Source: CAD feature listing. Evaluate the final solid. Frame: model axes, mm. Face numbers are marked on the shaded views. A direction names the side the tool comes from. Give positions to 0.01 mm unless a question says otherwise; leave off trailing zeros. Write each loop counter-clockwise with the first axis right and the second up, starting at its lowest first coordinate (ties: lowest second). Pieces come first, ordered by that corner, then holes. Notation, with made-up numbers: (-32, 84.25) -> (-12, 84.25) arc R26 ccw to (-12, 122.25) -> close; hole circle Ø10 at (-10, 84.5). An arc over 180 degrees is marked (long way). Use a Markdown table: item, result. Add a question column.
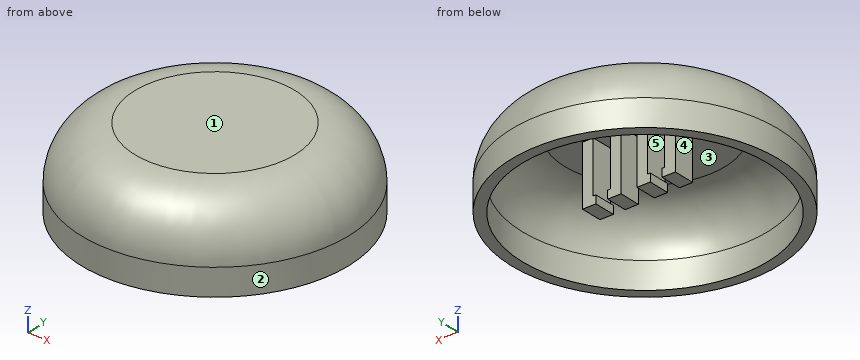
```python
from build123d import *

# Parameters (mm, degrees)
F0_R      = 31.75
F1_DEPTH  = 19.05
F2_R      = 12.7
F3_T      = -2.54
F5_W      = 2.54
F5_H      = 5.08
F6_DEPTH  = 14.224
F7_W      = 5.08
F7_H      = 1.905
F8_DEPTH  = 0.635
F9_W      = 5.08
F9_H      = 1.905
F10_DEPTH = 0.635
F11_W     = 5.08
F11_H     = 1.905
F12_DEPTH = 0.635
F13_W     = 5.08
F13_H     = 1.905
F14_DEPTH = 0.635


with BuildPart() as f1:
    # F0 (on Top) → F1 (new body)
    with BuildSketch(Plane.XY):
        Circle(F0_R)
    extrude(amount=F1_DEPTH)

    # F2
    f2_edges = [f1.edges().sort_by_distance(p)[0] for p in [
        (-31.75, 0, 19.05),
    ]]
    fillet(f2_edges, radius=F2_R)

    # F3
    f3_openings = [f1.faces().sort_by_distance(p)[0] for p in [
        (0, 0, 0),
    ]]
    offset(amount=F3_T, openings=f3_openings)

    # F5 (on face) → F6 (join)
    with BuildSketch(Plane(origin=(0, 0, 16.51), x_dir=(1, 0, 0), z_dir=(0, 0, -1))):
        with Locations((9.449818, -2.54)):
            Rectangle(F5_W, F5_H)
        with Locations((2.845818, -2.54)):
            Rectangle(F5_W, F5_H)
        with Locations((-3.48516, -2.54)):
            Rectangle(F5_W, F5_H)
        with Locations((-10.08916, -2.54)):
            Rectangle(F5_W, F5_H)
    extrude(amount=F6_DEPTH)

    # F7 (on face) → F8 (join)
    with BuildSketch(Plane(origin=(-4.75516, 0, 0), x_dir=(0, -1, 0), z_dir=(-1, 0, 0))):
        with Locations((-2.54, 3.2385)):
            Rectangle(F7_W, F7_H)
    extrude(amount=F8_DEPTH)

    # F9 (on face) → F10 (join)
    with BuildSketch(Plane.YZ.offset(4.115818)):
        with Locations((2.54, 3.2385)):
            Rectangle(F9_W, F9_H)
    extrude(amount=F10_DEPTH)

    # F11 (on face) → F12 (join)
    with BuildSketch(Plane(origin=(8.179818, 0, 0), x_dir=(0, -1, 0), z_dir=(-1, 0, 0))):
        with Locations((-2.54, 3.2385)):
            Rectangle(F11_W, F11_H)
    extrude(amount=F12_DEPTH)

    # F13 (on face) → F14 (join)
    with BuildSketch(Plane.YZ.offset(-8.81916)):
        with Locations((2.54, 3.2385)):
            Rectangle(F13_W, F13_H)
    extrude(amount=F14_DEPTH)


solid = f1.part
```
(1) First-contact query: pin 1 Ø5.5 at (y, z) = (2, 12.5) entering from -X; pin 2 Ø4 at (y, z) = (2.5, 8.5) entering from +X; pin 3 Ø5.5 at (y, z) = (1.5, 9.5) entering from -X. Flat tips, straight axial feed; report the tip coordinate or a pass-through.
(2) Cut plane C-C on x = 0. Return the cut outline in (y, z), then the cut area to 3 significant figures.
(3) Cut plane A-A on z = 12.25. Return the cut outline in (x, y), then the cut area to 3 significant figures.
(4) Mould query, pull axis Y, two halves, no side actions, for the marked faces 1, 2 and 3. Classes: +Y half, -Y half, draft (parallel to the pull), parting line (faces both ways), or undercut.
(5) Material intervals for L1, parallel to Y at x = 0, z = 2; L2, parallel to Y at x = 3, z = 7; L3, parallel to X at y = 23, z = 5.25, sorted ascending.
(6) Cut plane B-B on z = 15.5. Return the cut outline in (x, y).
(7) Access query for the marked faces 4 and 5. Directions: +Z, -Z, +X, -X, +Y, -Y. A direction counts if a zero-diameter tool reaches every point of the face in a straight line with its end or side. Return the directions, or none.
Output:
| question | item | result |
|---|---|---|
| 1 | pin 1 | x = -31.24 |
| 1 | pin 2 | x = 31.71 |
| 1 | pin 3 | x = -31.73 |
| 2 | outline | (-31.75, 0) -> (-29.21, 0) -> (-29.21, 6.35) arc R10.16 cw to (-19.05, 16.51) -> (19.05, 16.51) arc R10.16 cw to (29.21, 6.35) -> (29.21, 0) -> (31.75, 0) -> (31.75, 6.35) arc R12.7 ccw to (19.05, 19.05) -> (-19.05, 19.05) arc R12.7 ccw to (-31.75, 6.35) -> close |
| 2 | area | 220 mm^2 |
| 3 | outline | circle Ø60.59 at (0, 0); (-11.36, 0) -> (-8.82, 0) -> (-8.82, 5.08) -> (-11.36, 5.08) -> close; (-4.76, 0) -> (-2.22, 0) -> (-2.22, 5.08) -> (-4.76, 5.08) -> close; (1.58, 0) -> (4.12, 0) -> (4.12, 5.08) -> (1.58, 5.08) -> close; (8.18, 0) -> (10.72, 0) -> (10.72, 5.08) -> (8.18, 5.08) -> close; hole circle Ø54.64 at (0, 0) |
| 3 | area | 590 mm^2 |
| 4 | face 1 | draft |
| 4 | face 2 | parting line |
| 4 | face 3 | undercut |
| 5 | L1 | -31.75 to -29.21, 29.21 to 31.75 |
| 5 | L2 | -31.59 to -29.03, 0 to 5.08, 29.03 to 31.59 |
| 5 | L3 | -21.89 to -18.01, 18.01 to 21.89 |
| 6 | outline | circle Ø55.71 at (0, 0); (-11.36, 0) -> (-8.82, 0) -> (-8.82, 5.08) -> (-11.36, 5.08) -> close; (-4.76, 0) -> (-2.22, 0) -> (-2.22, 5.08) -> (-4.76, 5.08) -> close; (1.58, 0) -> (4.12, 0) -> (4.12, 5.08) -> (1.58, 5.08) -> close; (8.18, 0) -> (10.72, 0) -> (10.72, 5.08) -> (8.18, 5.08) -> close; hole circle Ø46.93 at (0, 0) |
| 7 | face 4 | -Z |
| 7 | face 5 | none |
